```python
from build123d import *

# Parameters (mm, degrees)
FILLET1_R = 0.5


with BuildPart() as part:
    # Sketch1 → Revolve1 (revolve)
    with BuildSketch(Plane.XY):
        with BuildLine():
            Line((-15.538461538, 10), (-25, 0))
            ThreePointArc((-25, 0), (-21.46926352, -12.809009482), (-11.874342087, -22))
            Line((-11.874342087, -22), (-5, -22))
            Line((-5, -22), (-5, -12))
            Line((-5, -12), (-2.5, -12))
            Line((-2.5, -12), (-2.5, 8))
            Line((-2.5, 8), (-12.7, 8))
            Line((-12.7, 8), (-12.7, 10))
            Line((-12.7, 10), (-15.538461538, 10))
        make_face()
    revolve(axis=Axis((0, 0, 0), (0, -1, 0)))

    # Fillet1
    fillet1_edges = [part.edges().sort_by_distance(p)[0] for p in [
        (5, -22, 0),
        (11.874342087, -22, 0),
    ]]
    fillet(fillet1_edges, radius=FILLET1_R)


solid = part.part
```
CAD build for the part. Positions are in the model's coordinates, mm. A direction names the side the tool comes from. Round coordinates to 2 decimals unless told otherwise and drop trailing zeros. Order: outer loops, then holes, each group sorted by start corner. A loop starts at its lowest first (then second) coordinate and runs counter-clockwise, first axis right, second up.
Item 1: Tool access for faces 1 (the face through (1.08, -16.68, 4.88)), 2 (the face through (2.75, 9.01, 12.4)), 3 (the face through (-13, 10, 0)): list every direction of +Z, -Z, +X, -X, +Y, -Y with a clear straight run to the whole face (end or side of a thin tool).
Item 2: Mould opens along X. For faces 4 (the face through (-5, -22, 3)), 5 (the face through (0.54, -1.86, 2.44)), 6 (the face through (2.1, 9.374, -15.993)) say: pulls with the +X half, pulls with the -X half, needs draft (parallel to the pull), parting line crosses it, or undercut.
Item 3: Probe line 1 along Y through (x, z) = (4, 0.5); line 2 along Y through (x, z) = (-5, 8); line 3 along Z through (x, y) = (0, 1). List the from-to ranges inside material, lowest first.
Item 4: Pin check, flat tips, straight feed: pin 1 (4 mm diameter, centred on x = -11.5, z = -17, fed in from +Y); pin 2 (3 mm diameter, centred on x = 16, y = -3, fed in from -Z); pin 3 (8 mm diameter, centred on x = 17.5, y = -11.5, fed in from +Z). Stop position of each tip, or through.
Item 5: Saw through at A-A on y = 6.5. Write the cut outline in (x, z).
Item 6: Saw through at B-B on y = -6.5. Write the cut outline in (x, z).
Reported:
1. face 1: -Y
1. face 2: +Y
1. face 3: +Z, -Z, +X, -X, +Y
2. face 4: needs draft
2. face 5: undercut
2. face 6: parting line crosses it
3. line 1: y = -12 to 8
3. line 2: y = -22 to 8
3. line 3: z = -24.05 to -2.5, 2.5 to 24.05
4. pin 1: stops at y = 6.84
4. pin 2: stops at z = -20.16
4. pin 3: stops at z = 18.39
5. outline: circle Ø37.7 at (0, 0); hole circle Ø5 at (0, 0)
6. outline: circle Ø48.28 at (0, 0); hole circle Ø5 at (0, 0)
